Source: CAD feature listing. Evaluate the final solid. Frame: model axes, mm. Face numbers are marked on the shaded views. A direction names the side the tool comes from. Give positions to 0.01 mm unless a question says otherwise; leave off trailing zeros. Order: outer loops, then holes, each group sorted by start corner. A loop starts at its lowest first (then second) coordinate and runs counter-clockwise, first axis right, second up.
```python
from build123d import *

# Parameters (mm, degrees)
SKETCH1_R           = 12.5
BOSS_EXTRUDE1_DEPTH = 1.5
SKETCH2_R           = 12.5
SKETCH2_R_2         = 0.75
BOSS_EXTRUDE2_DEPTH = 3
SKETCH3_R           = 1.25
CUT_EXTRUDE1_DEPTH  = 20.771458422
SKETCH4_R           = 12.5
SKETCH4_R_2         = 9.5
CUT_EXTRUDE2_DEPTH  = 1.5
SKETCH5_R           = 3
CUT_EXTRUDE3_DEPTH  = 1.5


with BuildPart() as part:
    # Sketch1 → Boss-Extrude1 (new body)
    with BuildSketch(Plane.XY):
        with Locations((0.807446417, 1.413031229)):
            Circle(SKETCH1_R)
        with BuildLine():
            Line((2.907446417, -2.065401928), (8.830836384, -1.541239144))
            ThreePointArc((8.830836384, -1.541239144), (9.200973023, -0.215222775), (9.353491615, 1.153009157))
            ThreePointArc((9.353491615, 1.153009157), (9.257446417, 1.413031229), (9.353491615, 1.673053302))
            ThreePointArc((9.353491615, 1.673053302), (9.200973023, 3.041285234), (8.830836384, 4.367301602))
            Line((8.830836384, 4.367301602), (2.907446417, 4.891464387))
            Line((2.907446417, 4.891464387), (2.907446417, 7.863031229))
            ThreePointArc((2.907446417, 7.863031229), (0.807446417, 9.963031229), (-1.292553583, 7.863031229))
            Line((-1.292553583, 7.863031229), (-1.292553583, 4.398412277))
            ThreePointArc((-1.292553583, 4.398412277), (-1.386241751, 4.330261461), (-1.477719845, 4.259171626))
            Line((-1.477719845, 4.259171626), (-7.361314725, 3.937678018))
            ThreePointArc((-7.361314725, 3.937678018), (-7.615427173, 2.881942556), (-7.733677844, 1.80251341))
            ThreePointArc((-7.733677844, 1.80251341), (-7.242553583, 1.413031229), (-7.733677844, 1.023549049))
            ThreePointArc((-7.733677844, 1.023549049), (-7.615427173, -0.055880097), (-7.361314725, -1.11161556))
            Line((-7.361314725, -1.11161556), (-1.477719845, -1.433109167))
            ThreePointArc((-1.477719845, -1.433109167), (-1.386241751, -1.504199002), (-1.292553583, -1.572349818))
            Line((-1.292553583, -1.572349818), (-1.292553583, -5.036968771))
            ThreePointArc((-1.292553583, -5.036968771), (0.807446417, -7.136968771), (2.907446417, -5.036968771))
            Line((2.907446417, -5.036968771), (2.907446417, -2.065401928))
        make_face(mode=Mode.SUBTRACT)
    extrude(amount=BOSS_EXTRUDE1_DEPTH)

    # Sketch2 → Boss-Extrude2 (add)
    with BuildSketch(Plane.XY.offset(1.5)):
        with Locations((0.807446417, 1.413031229)):
            Circle(SKETCH2_R)
        with Locations((0.807446417, 1.413031229)):
            Circle(SKETCH2_R_2, mode=Mode.SUBTRACT)
    extrude(amount=BOSS_EXTRUDE2_DEPTH)

    # Sketch3 → Cut-Extrude1 (cut, through all)
    with BuildSketch(Plane.XY.offset(4.5)):
        with Locations((7.171407447, 7.77699226)):
            Circle(SKETCH3_R)
        with Locations((7.171407447, -4.950929801)):
            Circle(SKETCH3_R)
        with Locations((-5.556514614, -4.950929801)):
            Circle(SKETCH3_R)
        with Locations((-5.556514614, 7.77699226)):
            Circle(SKETCH3_R)
    extrude(amount=-CUT_EXTRUDE1_DEPTH, mode=Mode.SUBTRACT)

    # Sketch4 → Cut-Extrude2 (cut)
    with BuildSketch(Plane(origin=(0, 0, 0), x_dir=(-1, 0, 0), z_dir=(0, 0, -1))):
        with Locations((-0.807446417, 1.413031229)):
            Circle(SKETCH4_R)
        with Locations((-0.807446417, 1.413031229)):
            Circle(SKETCH4_R_2, mode=Mode.SUBTRACT)
    extrude(amount=-CUT_EXTRUDE2_DEPTH, mode=Mode.SUBTRACT)

    # Sketch5 → Cut-Extrude3 (cut)
    with BuildSketch(Plane.XY.offset(4.5)):
        with Locations((0.807446417, 1.413031229)):
            Circle(SKETCH5_R)
    extrude(amount=-CUT_EXTRUDE3_DEPTH, mode=Mode.SUBTRACT)


solid = part.part
```
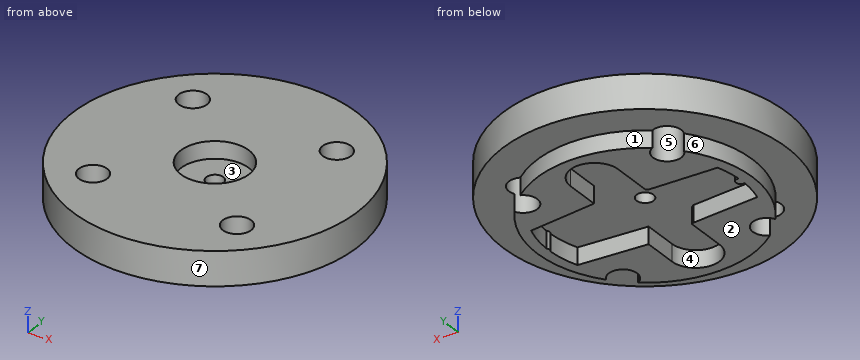
1) Reachability of the marked faces 1, 2, 3 and 4 from +Z, -Z, +X, -X, +Y, -Y: full face, straight path, thin tool, end or side. Return the list, or none.
Report:
face 1: -Z, +Y
face 2: -Z, +X, -X, +Y, -Y
face 3: +Z
face 4: -Z
2) Draft query along X for the marked faces 5, 6 and 7. Return one class per face: +X half, -X half, draft (parallel to the pull), parting line (faces both ways), or undercut.
Report:
face 5: undercut
face 6: -X half
face 7: parting line
3) Section query A-A, the plane z = 1. Return the cut outline in (x, y).
Report:
outline: (-6.69, -4.42) arc R1.25 cw (long way) to (-5.03, -6.08) arc R9.5 ccw to (6.64, -6.08) arc R1.25 cw (long way) to (8.3, -4.42) arc R9.5 ccw to (8.3, 7.25) arc R1.25 cw (long way) to (6.64, 8.91) arc R9.5 ccw to (-5.03, 8.91) arc R1.25 cw (long way) to (-6.69, 7.25) arc R9.5 ccw to start; hole (-7.73, 1.02) arc R8.55 ccw to (-7.36, -1.11) - (-1.48, -1.43) arc R3.65 ccw to (-1.29, -1.57) - (-1.29, -5.04) arc R2.1 ccw to (2.91, -5.04) - (2.91, -2.07) - (8.83, -1.54) arc R8.55 ccw to (9.35, 1.15) arc R0.4 cw to (9.35, 1.67) arc R8.55 ccw to (8.83, 4.37) - (2.91, 4.89) - (2.91, 7.86) arc R2.1 ccw to (-1.29, 7.86) - (-1.29, 4.4) arc R3.65 ccw to (-1.48, 4.26) - (-7.36, 3.94) arc R8.55 ccw to (-7.73, 1.8) arc R0.4 cw (long way) to start
4) Section query D-D, the plane z = 2.25. Return the cut outline in (x, y), and give its area (3 significant figures).
Report:
outline: circle Ø25 at (0.81, 1.41); hole circle Ø2.5 at (-5.56, -4.95); hole circle Ø2.5 at (-5.56, 7.78); hole circle Ø1.5 at (0.81, 1.41); hole circle Ø2.5 at (7.17, -4.95); hole circle Ø2.5 at (7.17, 7.78)
area: 469 mm2
5) Material intervals for L1, parallel to Y at x = 0.75, z = 2.9; L2, parallel to X at y = -6, z = 2.45; L3, parallel to Y at x = 1, z = 3.7, sorted ascending.
Report:
L1: y = -11.09 to 0.67, 2.16 to 13.91
L2: x = -9.26 to -6.24, -4.88 to 6.49, 7.85 to 10.87
L3: y = -11.09 to -1.58, 4.41 to 13.91
6) Pin query (flat end, axial travel): pin 1 (1.7 mm diameter, centred on x = 0.81, y = 1.41, fed in from +Z); pin 2 (1.6 mm diameter, centred on y = 5.5, z = 1, fed in from +X); pin 3 (1.5 mm diameter, centred on x = -5.56, y = -4.95, fed in from -Z); pin 4 (1.5 mm diameter, centred on y = -5.5, z = 1.5, fed in from -X). Return the tip coordinate at first contact, or that it passes through.
Report:
pin 1: stops at z = 3
pin 2: stops at x = 12.82
pin 3: passes through
pin 4: stops at x = -10.07
7) Section query B-B, the plane x = 3.5. Return the cut outline in (y, z), and give its area (3 significant figures).
Report:
outline: (-10.79, 1.5) - (-7.7, 1.5) - (-7.7, 0) - (-2.01, 0) - (-2.01, 1.5) - (4.84, 1.5) - (4.84, 0) - (10.52, 0) - (10.52, 1.5) - (13.62, 1.5) - (13.62, 4.5) - (2.74, 4.5) - (2.74, 3) - (0.09, 3) - (0.09, 4.5) - (-10.79, 4.5) - close
area: 86.3 mm2
8) Section query C-C, the plane y = 5.5. Return the cut outline in (x, z), and give its area (3 significant figures).
Report:
outline: (-11.01, 1.5) - (-7.77, 1.5) - (-7.77, 0) - (-1.29, 0) - (-1.29, 1.5) - (2.91, 1.5) - (2.91, 0) - (9.38, 0) - (9.38, 1.5) - (12.62, 1.5) - (12.62, 4.5) - (-11.01, 4.5) - close
area: 90.3 mm2
